Autodesk Inventor part; units mm, degrees
ref_plane "YZ Plane" through (0, 0, 0) normal (1, 0, 0) x (0, 1, 0)
ref_plane "XZ Plane" through (0, 0, 0) normal (0, 1, 0) x (-1, 0, 0)
ref_plane "XY Plane" through (0, 0, 0) normal (0, 0, 1) x (1, 0, 0)
sketch "Sketch1" plane through (0, 0, 0) normal (0, 0, 1) x (1, 0, 0)
  line L0 (0, 0) -> (508, 0)
  line L1 (508, 0) -> (508, 63.5)
  line L2 (508, 63.5) -> (0, 63.5)
  line L3 (0, 63.5) -> (0, 0)
  circle A0 centre (484.886, 31.75) radius 10.9982
  circle A1 centre (73.914, 53.3905) radius 3.175
  circle A2 centre (162.9664, 53.3905) radius 3.175
  circle A3 centre (252.0188, 53.3868) radius 3.175
  circle A4 centre (341.0712, 53.3868) radius 3.175
  circle A5 centre (430.1236, 53.3868) radius 3.175
  circle A6 centre (73.914, 8.9405) radius 3.175
  circle A7 centre (162.9664, 8.9368) radius 3.175
  circle A8 centre (252.0188, 8.9368) radius 3.175
  circle A9 centre (341.0712, 8.9368) radius 3.175
  circle A10 centre (430.1236, 8.9368) radius 3.175
  line L4 (61.214, 43.0781) -> (73.5873, 21.6469)
  line L5 (48.8407, 21.6469) -> (61.214, 43.0781)
  line L6 (137.414, 43.0781) -> (149.7873, 21.6469)
  line L7 (149.7873, 21.6469) -> (125.0407, 21.6469)
  line L8 (125.0407, 21.6469) -> (137.414, 43.0781)
  line L9 (99.314, 21.6469) -> (86.9407, 43.0781)
  line L10 (86.9407, 43.0781) -> (111.6873, 43.0781)
  line L11 (111.6873, 43.0781) -> (99.314, 21.6469)
  line L12 (26.7802, 38.1) -> (30.4463, 31.75)
  line L13 (30.4463, 31.75) -> (26.7681, 25.4)
  line L14 (26.7681, 25.4) -> (19.4478, 25.4)
  line L15 (19.4478, 25.4) -> (15.7817, 31.75)
  line L16 (15.7817, 31.75) -> (19.4478, 38.1)
  line L17 (19.4478, 38.1) -> (26.7802, 38.1)
  line L18 (48.8407, 21.6469) -> (73.5873, 21.6469)
  line L19 (289.4838, 43.0781) -> (301.8571, 21.6469)
  line L20 (301.8571, 21.6469) -> (277.1105, 21.6469)
  line L21 (277.1105, 21.6469) -> (289.4838, 43.0781)
  line L22 (263.7571, 43.0781) -> (251.3838, 21.6469)
  line L23 (251.3838, 21.6469) -> (239.0105, 43.0781)
  line L24 (239.0105, 43.0781) -> (263.7571, 43.0781)
  line L25 (213.2838, 43.0781) -> (225.6571, 21.6469)
  line L26 (200.9105, 21.6469) -> (225.6571, 21.6469)
  line L27 (200.9105, 21.6469) -> (213.2838, 43.0781)
  line L28 (441.5536, 43.0781) -> (453.9269, 21.6469)
  line L29 (453.9269, 21.6469) -> (429.1803, 21.6469)
  line L30 (429.1803, 21.6469) -> (441.5536, 43.0781)
  line L31 (415.8269, 43.0781) -> (403.4536, 21.6469)
  line L32 (403.4536, 21.6469) -> (391.0803, 43.0781)
  line L33 (391.0803, 43.0781) -> (415.8269, 43.0781)
  line L34 (365.3536, 43.0781) -> (377.7269, 21.6469)
  line L35 (352.9803, 21.6469) -> (377.7269, 21.6469)
  line L36 (352.9803, 21.6469) -> (365.3536, 43.0781)
  line L37 (175.5175, 21.6469) -> (163.1442, 43.0781)
  line L38 (163.1442, 43.0781) -> (187.8909, 43.0781)
  line L39 (187.8909, 43.0781) -> (175.5175, 21.6469)
  line L40 (339.9607, 43.0781) -> (327.5873, 21.6469)
  line L41 (327.5873, 21.6469) -> (315.214, 43.0781)
  line L42 (315.214, 43.0781) -> (339.9607, 43.0781)
  point P0 (135.1884, 47.8306)
  point P1 (135.1884, 33.5431)
  point P2 (23.114, 19.05)
  point P3 (23.114, 25.4)
  point P4 (287.2582, 33.5431)
  point P5 (439.328, 33.5431)
  dimension "d18" = 44.45
  dimension "d36" = 56.5658
  dimension "d69" = 126.3396
  dimension "d72" = 25.4
  dimension "d0" = 508
  dimension "d1" = 63.5
  dimension "d3" = 21.9964
  dimension "d12" = 6.35
  dimension "d15" = 89.0524
  dimension "d44" = 6.35
  dimension "d66" = 100.9467
  dimension "d91" = 22.0726
  dimension "d97" = 152.0698
  dimension "d102" = 51.1231
extrude "Extrusion1" add sketch "Sketch1" along normal blind 12.7 contours L3 L2 L1 L0 | L4 L18 L5 | L12 L13 L14 L15 L16 L17 | L19 L20 L21 | L22 L23 L24 | L25 L26 L27 | L28 L29 L30 | L31 L32 L33 | L34 L35 L36 | L37 L38 L39 | L40 L41 L42
extrude "Extrusion2" cut sketch "Sketch1" along normal blind 25.4 contours L12 L13 L14 L15 L16 L17
extrude "Extrusion4" cut sketch "Sketch1" along normal blind 12.7 contours L4 L18 L5
extrude "Extrusion5" cut sketch "Sketch1" along normal blind 12.7 contours L19 L20 L21 | L22 L23 L24 | L25 L26 L27 | L28 L29 L30 | L31 L32 L33 | L34 L35 L36 | L37 L38 L39 | L40 L41 L42
properties part number "arm_plate_btw_support_bicep"
Here's how the part is built. I have some questions about the finished solid (model axes, mm). Round coordinates to 2 decimals unless told otherwise and drop trailing zeros. Answer in a Markdown table with one row per item.
Item 1: Thinking about a two-plate mould opening in X: for faces 1 (the face through (508, 31, 6)), 2 (the face through (258, 63.5, 6)), 3 (the face through (495.376, 28.446, 6.261)), which applies, +X half, -X half, draft (parallel to the pull), parting line (faces both ways), or undercut?
A:
| item | result |
|---|---|
| face 1 | +X half |
| face 2 | draft |
| face 3 | undercut |
Item 2: I'm going to push flat-ended pins straight in: pin 1 (1 mm diameter, centred on x = 364, y = 56, fed in from -Z); pin 2 (5.5 mm diameter, centred on x = 162.97, y = 8.94, fed in from -Z). Where does each tip first touch, or does it pass through?
A:
| item | result |
|---|---|
| pin 1 | stops at z = 0 |
| pin 2 | passes through |
Item 3: Imagine slicing it at A-A, the plane z = 5.5. State how many separate pieces and enclosed holes the cut face has, and give its area (3 significant figures).
A:
| item | result |
|---|---|
| separate pieces | 1 |
| enclosed holes | 23 |
| area | 28,500 mm2 |
Item 4: If I drill on L1, parallel to Y at x = 341, z = 5.75; L2, parallel to Y at x = 76, z = 5.25; L3, parallel to X at y = 8, z = 6.5, over which ranges is the centre line in solid material (lowest first)? Write a range as from..to.
A:
| item | result |
|---|---|
| L1 | y = 0..5.76, 12.11..50.21, 56.56..63.5 |
| L2 | y = 0..6.55, 11.33..51, 55.78..63.5 |
| L3 | x = 0..70.88, 76.95..159.93, 166..248.99, 255.05..338.04, 344.1..427.09, 433.16..508 |
